Work out the finished part from the listing and answer in its coordinate system (mm). A direction names the side the tool comes from. Give positions to 0.01 mm unless a question says otherwise; leave off trailing zeros. Order: outer loops, then holes, each group sorted by start corner. A loop starts at its lowest first (then second) coordinate and runs counter-clockwise, first axis right, second up. Notation, with made-up numbers: (-30.5, 60) - (-12.5, 60) arc R27 ccw to (-12.5, 84) - close; hole circle Ø9 at (30.25, -31). An arc over 180 degrees is marked (long way). Put each result on its own line as item: value.
```python
from build123d import *

# Parameters (mm, degrees)
F1_DEPTH = 63.5
F2_DEPTH = 6.35
F3_DEPTH = 22.225
F4_DEPTH = 2.286
F5_R     = 6.35


with BuildPart() as f1:
    # F0 (on Front) → F1 (new body, symmetric)
    with BuildSketch(Plane.XZ):
        Polygon((41.275, -9.525), (41.275, 9.525), (-3.175, 9.525), (-41.275, 9.525), (-41.275, -9.525), align=None)
    extrude(amount=F1_DEPTH, both=True)

    # F0 (on Front) → F2 (join, symmetric)
    with BuildSketch(Plane.XZ):
        with BuildLine():
            Line((-3.175, 9.525), (41.275, 9.525))
            Line((41.275, 9.525), (41.275, 54.246902))
            ThreePointArc((41.275, 54.246902), (45.92468, 65.472222), (57.15, 70.121902))
            Line((57.15, 70.121902), (57.320657, 70.121902))
            Line((57.320657, 70.121902), (57.320657, 90.37864))
            add(Edge.make_bspline(
                [(-1.011012, 70.259469), (16.740772, 82.473388), (37.932847, 90.39046), (57.320657, 90.37864)],
                knots=[71.739647, 71.739647, 71.739647, 71.739647, 127.508489, 127.508489, 127.508489, 127.508489], degree=3))
            ThreePointArc((-1.011012, 70.259469), (-2.631555, 62.325967), (-3.175, 54.246902))
            Line((-3.175, 54.246902), (-3.175, 9.525))
        make_face()
    extrude(amount=F2_DEPTH, both=True)

    # F0 (on Front) → F3 (join, symmetric)
    with BuildSketch(Plane.XZ):
        Polygon((57.320657, 90.37864), (57.320657, 70.121902), (57.320657, 61.80364), (108.120657, 61.80364), (108.120657, 90.37864), align=None)
    extrude(amount=F3_DEPTH, both=True)

    # F0 (on Front) → F4 (join)
    with BuildSketch(Plane.XZ):
        with BuildLine():
            Line((-41.275, 9.525), (-3.175, 9.525))
            Line((-3.175, 9.525), (-3.175, 54.246902))
            ThreePointArc((-3.175, 54.246902), (-2.631555, 62.325967), (-1.011012, 70.259469))
            add(Edge.make_bspline(
                [(-41.275, 9.525), (-40.989055, 31.725856), (-23.846463, 54.547789), (-1.011012, 70.259469)],
                knots=[0, 0, 0, 0, 71.739647, 71.739647, 71.739647, 71.739647], degree=3))
        make_face()
    extrude(amount=F4_DEPTH)

    # F5
    f5_edges = [f1.edges().sort_by_distance(p)[0] for p in [
        (41.275, 63.5, 0),
        (-41.275, 63.5, 0),
        (41.275, -63.5, 0),
        (-41.275, -63.5, 0),
        (41.275, 0, -9.525),
    ]]
    fillet(f5_edges, radius=F5_R)


solid = f1.part
```
(1) Section D-D, the plane x = 96 is taken. Write down the section's boundary in (y, z) (3 decimals).
Geometry check:
outline: (-22.225, 61.804) - (22.225, 61.804) - (22.225, 90.379) - (-22.225, 90.379) - close
(2) Straight lines are drawn through the part: line 1 (Z direction, x = 34, y = 13) (3 decimals); line 2 (Z direction, x = 89, y = -18.5); line 3 (Y direction, x = -34, z = 26.5). For each, find the intervals that lie inside material, in ascending order.
Geometry check:
line 1: z = -9.525 to 9.525
line 2: z = 61.8 to 90.38
line 3: y = -2.29 to 0
(3) Given pin 1 (2 mm diameter, centred on x = 4.5, z = 35, fed in from -Y); pin 2 (1.5 mm diameter, centred on x = 3, z = 39, fed in from +Y); pin 3 (8 mm diameter, centred on y = -24.5, z = 14, fed in from -X); pin 4 (2 mm diameter, centred on y = -3.5, z = 22.5, fed in from -X) (3 decimals), each flat-ended and moving along its own axis, determine where each tip first touches the part or whether it passes through.
Geometry check:
pin 1: stops at y = -6.35
pin 2: stops at y = 6.35
pin 3: passes through
pin 4: stops at x = -3.175
(4) Section A-A, the plane y = -9.5 is taken. Write down the section's boundary in (x, z) (3 decimals), then the cut area to 3 significant figures.
Geometry check:
outline: (-41.275, -9.525) - (34.925, -9.525) arc R6.35 ccw to (41.275, -3.175) - (41.275, 9.525) - (-41.275, 9.525) - close; (57.321, 61.804) - (108.121, 61.804) - (108.121, 90.379) - (57.321, 90.379) - close
area: 3,020 mm²
(5) A tool of negligible diameter and unlimited length cuts with its end or side. For faces 1 (the face through (-4, -1, -9.525)), 2 (the face through (27, 6.35, 51)), 3 (the face through (82, 0, 61.804)), 4 (the face through (45.802, -0.089, 65.348)), 5 (the face through (-3.175, -4, 32)), from which of +Z, -Z, +X, -X, +Y, -Y can it reach the whole face along a straight path? Write none if from no direction.
Geometry check:
face 1: -Z, +X, -X, +Y, -Y
face 2: +Z, -X, +Y
face 3: -Z, +X, +Y, -Y
face 4: -Z, +Y, -Y
face 5: +Z, -X, -Y
(6) Section C-C, the plane y = 53 is taken. Write down the section's boundary in (x, z) (3 decimals).
Geometry check:
outline: (-41.275, -9.525) - (34.925, -9.525) arc R6.35 ccw to (41.275, -3.175) - (41.275, 9.525) - (-41.275, 9.525) - close
(7) Determine the mould class of faces 6 (the face through (-3.175, 3, 32)), 7 (the face through (-17, 0, 34)), 8 (the face through (57.321, -0.3, 69.9)), 9 (the face through (39.365, -61.689, 0.133)) for opening direction X: pulls with the +X half, pulls with the -X half, needs draft (parallel to the pull), parting line crosses it, or undercut.
Geometry check:
face 6: pulls with the -X half
face 7: needs draft
face 8: undercut
face 9: pulls with the +X half
(8) Section B-B, the plane z = 7.5 is taken. Write down the section's boundary in (x, y) (3 decimals).
Geometry check:
outline: (-41.275, -57.15) arc R6.35 ccw to (-34.925, -63.5) - (34.925, -63.5) arc R6.35 ccw to (41.275, -57.15) - (41.275, 57.15) arc R6.35 ccw to (34.925, 63.5) - (-34.925, 63.5) arc R6.35 ccw to (-41.275, 57.15) - close
